```python
from build123d import *

# Parameters (mm, degrees)
SKETCH1_R           = 2.1
BOSS_EXTRUDE1_DEPTH = 383.54
CHAMFER1_SIZE       = 0.2828


with BuildPart() as part:
    # Sketch1 → Boss-Extrude1 (new body)
    with BuildSketch(Plane.XY):
        Polygon((-3, 8), (-3, 10), (-10, 10), (-10, 3), (-8, 3), (-8, 6), (-7, 6), (-4, 3), (-4, -3), (-7, -6), (-8, -6), (-8, -3), (-10, -3), (-10, -10), (-3, -10), (-3, -8), (-6, -8), (-6, -7), (-3, -4), (3, -4), (6, -7), (6, -8), (3, -8), (3, -10), (10, -10), (10, -3), (8, -3), (8, -6), (7, -6), (4, -3), (4, 3), (7, 6), (8, 6), (8, 3), (10, 3), (10, 10), (3, 10), (3, 8), (6, 8), (6, 7), (3, 4), (-3, 4), (-6, 7), (-6, 8), align=None)
        Circle(SKETCH1_R, mode=Mode.SUBTRACT)
    extrude(amount=BOSS_EXTRUDE1_DEPTH)

    # Chamfer1
    chamfer1_edges = [part.edges().sort_by_distance(p)[0] for p in [
        (-8, -3, 191.77),
        (-8, 3, 191.77),
        (-10, 3, 191.77),
        (-10, 10, 191.77),
        (-3, 10, 191.77),
        (-3, 8, 191.77),
        (3, 8, 191.77),
        (3, 10, 191.77),
        (10, 10, 191.77),
        (10, 3, 191.77),
        (8, 3, 191.77),
        (8, -3, 191.77),
        (10, -3, 191.77),
        (10, -10, 191.77),
        (3, -10, 191.77),
        (3, -8, 191.77),
        (-3, -8, 191.77),
        (-3, -10, 191.77),
        (-10, -10, 191.77),
        (-10, -3, 191.77),
    ]]
    chamfer(chamfer1_edges, length=CHAMFER1_SIZE)


solid = part.part
```
CAD build for the part. Positions are in the model's coordinates, mm. A direction names the side the tool comes from. Round coordinates to 2 decimals unless told otherwise and drop trailing zeros.
Q1. Drop flat-ended pins along their axis: pin 1 (5 mm diameter, centred on x = 1, z = 233.5, fed in from +Y); pin 2 (1.8 mm diameter, centred on y = 0.5, z = 113, fed in from +X); pin 3 (5 mm diameter, centred on x = 0, z = 217, fed in from -Y). Give the stop position or say it passes through.
Q2. Two-plate mould, pull along X, no slides. Class faces 1 (the flat face through (-4, 0, 189)), 2 (the flat face through (-0.1, 2.4, 0)), 3 (the flat face through (4, 0, 189)), 4 (the flat face through (0, 4, 189)): pulls with the +X half, pulls with the -X half, needs draft (parallel to the pull), parting line crosses it, or undercut.
Q3. Wall check: L1, parallel to Y at x = 0, z = 303.5; L2, parallel to X at y = 7.25, z = 309; L3, parallel to Y at x = 8.75, z = 20. Give the ranges that are in metal, low to high.
Q4. Which spindle directions (+Z, -Z, +X, -X, +Y, -Y) get a long thin tool onto all of the face, cutting with end or side? Do faces 5 (the flat face through (0, -4, 189)), 6 (the flat face through (-6, 10, 189)). Say none if no direction does.
Results below:
1. pin 1: stops at y = 10
1. pin 2: stops at x = 4
1. pin 3: stops at y = -4
2. face 1: pulls with the -X half
2. face 2: needs draft
2. face 3: pulls with the +X half
2. face 4: undercut
3. L1: y = -4 to -2.1, 2.1 to 4
3. L2: x = -10 to -6, 6 to 10
3. L3: y = -10 to -3, 3 to 10
4. face 5: +Z, -Z, -Y
4. face 6: +Z, -Z, +X, -X, +Y
